Can you work these out from the model? Positions are in its coordinate system, mm. A direction names the side the tool comes from. Coordinates: 2 decimals unless noted, no trailing zeros. Order: outer loops, then holes, each group sorted by start corner. A loop starts at its lowest first (then second) coordinate and runs counter-clockwise, first axis right, second up. Notation, with made-up numbers: (-27.5, 66.25) -> (-14.5, 66.25) arc R26 cw to (-14.5, 101.25) -> close; hole circle Ø3 at (-7.5, -5). An arc over 180 degrees is marked (long way). Answer as a JSON object with one key per item and string values. Group by question number.
(1) If we mould it in two halves opening along Z, with no side actions, what happens to faces 4 (the flat face through (0, 0, 16)), 5 (the flat face through (-30, 0, 7)), 6 (the flat face through (29.01, 9.39, 10.4))? For each: pulls with the +Z half, pulls with the -Z half, needs draft (parallel to the pull), parting line crosses it, or undercut.
(2) I want a section at A-A, the plane y = -3.5. List the corners of the cut face in (x, z) for me.
(3) I need wall thicknesses on line 1 (X direction, y = 2, z = 6.75); line 2 (Z direction, x = -16.5, y = -1); line 3 (Z direction, x = -12.5, y = 12.25). Which ranges of each line are inside material? Lowest first, please.
(4) I want a section at C-C, the plane z = 13.75. List the corners of the cut face in (x, y) for me.
(5) I want a section at D-D, the plane y = 11.25. List the corners of the cut face in (x, z) for me.
(6) I want a section at B-B, the plane x = -8. List the corners of the cut face in (y, z) for me.
(7) Which directions (+Z, -Z, +X, -X, +Y, -Y) give clear straight access to the entire face, cutting with the end or side of a thin tool? Please do faces 1 (the flat face through (0, 1, 3)), 2 (the flat face through (0, 5, 17)), 3 (the flat face through (0.42, -10.73, 10.395)).
(8) For pin 1 (0.6 mm diameter, centred on x = 10, z = 17.5, fed in from +Y); pin 2 (1.5 mm diameter, centred on x = -19.5, z = 5.5, fed in from +Y); pin 3 (3 mm diameter, centred on x = 3, z = 7.5, fed in from -Y), each with a flat end and sliding along its axis, tell me the tip position at first contact or that it passes through.
from build123d import *

# Parameters (mm, degrees)
F0_W      = 60
F0_H      = 30
F1_DEPTH  = 3
F2_W      = 15
F2_H      = 15
F3_DEPTH  = 60
F4_W      = 5
F4_H      = 15
F5_DEPTH  = 60
F7_DEPTH  = 60
F9_DEPTH  = 58
F11_DEPTH = 2
F13_DEPTH = 2
F15_DEPTH = 2
F16_W     = 1.339746
F16_H     = 3
F17_DEPTH = 60


with BuildPart() as f1:
    # F0 (on Top) → F1 (new body)
    with BuildSketch(Plane.XY):
        Rectangle(F0_W, F0_H)
    extrude(amount=F1_DEPTH)

    # F2 (on face) → F3 (join)
    with BuildSketch(Plane.YZ.offset(30)):
        with Locations((-7.5, 10.5)):
            Rectangle(F2_W, F2_H)
    extrude(amount=-F3_DEPTH)

    # F4 (on face) → F5 (join)
    with BuildSketch(Plane.YZ.offset(30)):
        with Locations((2.5, 10.5)):
            Rectangle(F4_W, F4_H)
    extrude(amount=-F5_DEPTH)

    # F6 (on face) → F7 (cut, through all)
    with BuildSketch(Plane.YZ.offset(30)):
        Polygon((-15, 18), (-15, 3), (-6.339746, 18), align=None)
    extrude(amount=-F7_DEPTH, mode=Mode.SUBTRACT)

    # F8 (on face) → F9 (cut)
    with BuildSketch(Plane(origin=(-30, 0, 0), x_dir=(0, -1, 0), z_dir=(-1, 0, 0))):
        Polygon((-5, 16), (-5, 3), (12.690599, 3), (5.185045, 16), align=None)
    extrude(amount=-F9_DEPTH, mode=Mode.SUBTRACT)

    # F10 (on face) → F11 (join)
    with BuildSketch(Plane(origin=(-30, 0, 0), x_dir=(0, -1, 0), z_dir=(-1, 0, 0))):
        Polygon((6.339746, 18), (-5, 18), (-5, 16), (5.185045, 16), (12.690599, 3), (-5, 3), (-5, 0), (15, 0), (15, 3), align=None)
        Polygon((5.185045, 16), (-5, 16), (-5, 3), (12.690599, 3), align=None)
    extrude(amount=-F11_DEPTH)

    # F12 (on face) → F13 (join)
    with BuildSketch(Plane(origin=(-30, 0, 0), x_dir=(0, -1, 0), z_dir=(-1, 0, 0))):
        Polygon((-5, 3), (-5, 18), (-13.660254, 3), align=None)
        Polygon((6.339746, 18), (-5, 18), (-5, 3), (-13.660254, 3), (-15, 3), (-15, 0), (15, 0), (15, 3), align=None)
    extrude(amount=-F13_DEPTH)

    # F14 (on face) → F15 (join)
    with BuildSketch(Plane.YZ.offset(30)):
        Polygon((5, 3), (5, 18), (-6.339746, 18), (-15, 3), (-15, 0), (15, 0), (15, 3), (13.660254, 3), align=None)
        Polygon((13.660254, 3), (5, 18), (5, 3), align=None)
    extrude(amount=-F15_DEPTH)

    # F16 (on face) → F17 (cut)
    with BuildSketch(Plane.YZ.offset(30)):
        with Locations((14.330127, 1.5)):
            Rectangle(F16_W, F16_H)
    extrude(amount=-F17_DEPTH, mode=Mode.SUBTRACT)


solid = f1.part
Computed values:
{
 "1": {"face 4": "undercut", "face 5": "needs draft", "face 6": "pulls with the +Z half"},
 "2": {"outline": "(-30, 0) -> (30, 0) -> (30, 18) -> (-30, 18) -> close; hole (-28, 3) -> (28, 3) -> (28, 16) -> (-28, 16) -> close"},
 "3": {"line 1": "x = -30 to -28, 28 to 30", "line 2": "z = 0 to 3, 16 to 18", "line 3": "z = 0 to 3"},
 "4": {"outline": "(-30, -8.79) -> (30, -8.79) -> (30, 7.45) -> (28, 7.45) -> (28, -6.48) -> (-28, -6.48) -> (-28, 7.45) -> (-30, 7.45) -> close"},
 "5": {"outline": "(-30, 0) -> (30, 0) -> (30, 7.17) -> (28, 7.17) -> (28, 3) -> (-28, 3) -> (-28, 7.17) -> (-30, 7.17) -> close"},
 "6": {"outline": "(-15, 0) -> (13.66, 0) -> (13.66, 3) -> (-12.69, 3) -> (-5.19, 16) -> (5, 16) -> (5, 18) -> (-6.34, 18) -> (-15, 3) -> close"},
 "7": {"face 1": "+Y", "face 2": "+Z, +Y", "face 3": "+Z, +X, -X, -Y"},
 "8": {"pin 1": "stops at y = 5", "pin 2": "stops at y = -10.81", "pin 3": "stops at y = -13.27"}
}
